```python
from build123d import *

# Parameters (mm, degrees)
SKETCH_1_W          = 40
SKETCH_1_H          = 20
EXTRUDE_1_DEPTH     = 3
EXTRUDE_2_DEPTH     = 3
SKETCH_3_R          = 3
CUT_EXTRUDE_1_DEPTH = 3
SKETCH_4_W          = 40
SKETCH_4_H          = 15
SKETCH_4_R          = 3
EXTRUDE_3_DEPTH     = 3
FILLET_3_R          = 1.5
SKETCH_5_R          = 5
SKETCH_5_R_2        = 3
EXTRUDE_4_DEPTH     = 3
FILLET_4_R          = 1.5
CUT_EXTRUDE_2_DEPTH = 10
FILLET_6_R          = 0.5
CUT_EXTRUDE_3_DEPTH = 3


with BuildPart() as part:
    # 草图1 → 凸台-拉伸1 (new body)
    with BuildSketch(Plane.XY):
        Rectangle(SKETCH_1_W, SKETCH_1_H)
    extrude(amount=EXTRUDE_1_DEPTH)

    # 草图2 → 凸台-拉伸2 (add)
    with BuildSketch(Plane.XY.offset(3)):
        Polygon((-6.9, 8.2), (-6.9, 10), (-13.1, 10), (-13.1, 8.2), (-15.5, 8.2), (-15.5, 6.560660172), (-12.839339828, 3.9), (-7.160660172, 3.9), (-4.5, 6.560660172), (-4.5, 8.2), align=None)
        Polygon((-16.560660172, 5.5), (-18.2, 5.5), (-18.2, 3.1), (-20, 3.1), (-20, -3.1), (-18.2, -3.1), (-18.2, -5.5), (-16.560660172, -5.5), (-13.9, -2.839339828), (-13.9, 2.839339828), align=None)
        Polygon((-12.839339828, -3.9), (-7.160660172, -3.9), (-4.5, -6.560660172), (-4.5, -8.2), (-6.9, -8.2), (-6.9, -10), (-13.1, -10), (-13.1, -8.2), (-15.5, -8.2), (-15.5, -6.560660172), align=None)
        Polygon((18.2, 3.1), (20, 3.1), (20, -3.1), (18.2, -3.1), (18.2, -5.5), (16.560660172, -5.5), (13.9, -2.839339828), (13.9, 2.839339828), (16.560660172, 5.5), (18.2, 5.5), align=None)
        Polygon((13.1, 8.2), (13.1, 10), (6.9, 10), (6.9, 8.2), (4.5, 8.2), (4.5, 6.560660172), (7.160660172, 3.9), (12.839339828, 3.9), (15.5, 6.560660172), (15.5, 8.2), align=None)
        Polygon((7.160660172, -3.9), (12.839339828, -3.9), (15.5, -6.560660172), (15.5, -8.2), (13.1, -8.2), (13.1, -10), (6.9, -10), (6.9, -8.2), (4.5, -8.2), (4.5, -6.560660172), align=None)
    extrude(amount=EXTRUDE_2_DEPTH)

    # 草图3 → 切除-拉伸1 (cut)
    with BuildSketch(Plane(origin=(0, 0, 0), x_dir=(-1, 0, 0), z_dir=(0, 0, -1))):
        with Locations((-10, 0)):
            Circle(SKETCH_3_R)
        with Locations((10, 0)):
            Circle(SKETCH_3_R)
    extrude(amount=-CUT_EXTRUDE_1_DEPTH, mode=Mode.SUBTRACT)

    # 草图4 → 凸台-拉伸3 (add)
    with BuildSketch(Plane(origin=(0, 0, 0), x_dir=(-1, 0, 0), z_dir=(0, 0, -1))):
        with Locations((0, 17.5)):
            Rectangle(SKETCH_4_W, SKETCH_4_H)
        with Locations((-10, 19)):
            Circle(SKETCH_4_R, mode=Mode.SUBTRACT)
        with Locations((10, 19)):
            Circle(SKETCH_4_R, mode=Mode.SUBTRACT)
    extrude(amount=-EXTRUDE_3_DEPTH)

    # 圆角3
    fillet_3_edges = [part.edges().sort_by_distance(p)[0] for p in [
        (20, 25, 1.5),
        (-20, 25, 1.5),
        (20, -10, 1.5),
        (-20, -10, 1.5),
    ]]
    fillet(fillet_3_edges, radius=FILLET_3_R)

    # 草图5 → 凸台-拉伸4 (add)
    # profile 1 of 2: a face of its own
    with BuildSketch(Plane.XY.offset(3)):
        with Locations(Location((-10, 19, 0), (0, 0, 180))):
            Circle(SKETCH_5_R)
        with Locations(Location((-10, 19, 0), (0, 0, 180))):
            Circle(SKETCH_5_R_2, mode=Mode.SUBTRACT)
    # profile 2 of 2: a face of its own
    with BuildSketch(Plane.XY.offset(3)):
        with Locations(Location((10, 19, 0), (0, 0, 180))):
            Circle(SKETCH_5_R)
        with Locations(Location((10, 19, 0), (0, 0, 180))):
            Circle(SKETCH_5_R_2, mode=Mode.SUBTRACT)
    extrude(amount=EXTRUDE_4_DEPTH)

    # 圆角4
    fillet_4_edges = [part.edges().sort_by_distance(p)[0] for p in [
        (-5, 19, 3),
        (15, 19, 3),
    ]]
    fillet(fillet_4_edges, radius=FILLET_4_R)

    # 草图6 → 切除-拉伸2 (cut)
    with BuildSketch(Plane(origin=(0, 0, 0), x_dir=(-1, 0, 0), z_dir=(0, 0, -1))):
        Polygon((0, 23.005790595), (4, 23.005790595), (4, 25), (-4, 25), (-4, 23.005790595), align=None)
        Polygon((0, 15.005790595), (-4, 15.005790595), (-4, 12.005790595), (4, 12.005790595), (4, 15.005790595), align=None)
    extrude(amount=-CUT_EXTRUDE_2_DEPTH, mode=Mode.SUBTRACT)

    # 圆角6
    fillet_6_edges = [part.edges().sort_by_distance(p)[0] for p in [
        (4, 25, 1.5),
        (-4, 25, 1.5),
        (-4, 23.005790595, 1.5),
        (4, 23.005790595, 1.5),
        (4, 12.005790595, 1.5),
        (4, 15.005790595, 1.5),
        (-4, 15.005790595, 1.5),
        (-4, 12.005790595, 1.5),
    ]]
    fillet(fillet_6_edges, radius=FILLET_6_R)

    # 草图7 → 切除-拉伸3 (cut)
    with BuildSketch(Plane.XY.offset(6)):
        Polygon((-18.2, -3.1), (-18.2, -5.5), (-16.560660172, -5.5), (-13.9, -2.839339828), (-13.9, 2.839339828), (-16.560660172, 5.5), (-18.2, 5.5), (-18.2, 3.1), (-20, 3.1), (-20, 2.7), (-19.6, 2.7), (-17.8, 2.7), (-17.8, 5.1), (-16.726345597, 5.1), (-14.3, 2.673654403), (-14.3, -2.673654403), (-16.726345597, -5.1), (-17.8, -5.1), (-17.8, -2.7), (-19.6, -2.7), (-20, -2.7), (-20, -3.1), align=None)
        Polygon((-12.839339828, -3.9), (-15.5, -6.560660172), (-15.5, -8.2), (-13.1, -8.2), (-13.1, -10), (-12.7, -10), (-12.7, -9.6), (-12.7, -7.8), (-15.1, -7.8), (-15.1, -6.726345597), (-12.673654403, -4.3), (-7.326345597, -4.3), (-4.9, -6.726345597), (-4.9, -7.8), (-7.3, -7.8), (-7.3, -9.6), (-7.3, -10), (-6.9, -10), (-6.9, -8.2), (-4.5, -8.2), (-4.5, -6.560660172), (-7.160660172, -3.9), align=None)
        Polygon((-4.5, 8.2), (-6.9, 8.2), (-6.9, 10), (-7.3, 10), (-7.3, 9.6), (-7.3, 7.8), (-4.9, 7.8), (-4.9, 6.726345597), (-7.326345597, 4.3), (-12.673654403, 4.3), (-15.1, 6.726345597), (-15.1, 7.8), (-12.7, 7.8), (-12.7, 9.6), (-12.7, 10), (-13.1, 10), (-13.1, 8.2), (-15.5, 8.2), (-15.5, 6.560660172), (-12.839339828, 3.9), (-7.160660172, 3.9), (-4.5, 6.560660172), align=None)
        Polygon((15.5, 8.2), (13.1, 8.2), (13.1, 10), (12.7, 10), (12.7, 9.6), (12.7, 7.8), (15.1, 7.8), (15.1, 6.726345597), (12.673654403, 4.3), (7.326345597, 4.3), (4.9, 6.726345597), (4.9, 7.8), (7.3, 7.8), (7.3, 9.6), (7.3, 10), (6.9, 10), (6.9, 8.2), (4.5, 8.2), (4.5, 6.560660172), (7.160660172, 3.9), (12.839339828, 3.9), (15.5, 6.560660172), align=None)
        Polygon((18.2, 3.1), (18.2, 5.5), (16.560660172, 5.5), (13.9, 2.839339828), (13.9, -2.839339828), (16.560660172, -5.5), (18.2, -5.5), (18.2, -3.1), (20, -3.1), (20, -2.7), (19.6, -2.7), (17.8, -2.7), (17.8, -5.1), (16.726345597, -5.1), (14.3, -2.673654403), (14.3, 2.673654403), (16.726345597, 5.1), (17.8, 5.1), (17.8, 2.7), (19.6, 2.7), (20, 2.7), (20, 3.1), align=None)
        Polygon((7.160660172, -3.9), (4.5, -6.560660172), (4.5, -8.2), (6.9, -8.2), (6.9, -10), (7.3, -10), (7.3, -9.6), (7.3, -7.8), (4.9, -7.8), (4.9, -6.726345597), (7.326345597, -4.3), (12.673654403, -4.3), (15.1, -6.726345597), (15.1, -7.8), (12.7, -7.8), (12.7, -9.6), (12.7, -10), (13.1, -10), (13.1, -8.2), (15.5, -8.2), (15.5, -6.560660172), (12.839339828, -3.9), align=None)
    extrude(amount=-CUT_EXTRUDE_3_DEPTH, mode=Mode.SUBTRACT)


solid = part.part
```
The model under review builds one solid part; all positions refer to its coordinate system, in mm. A direction names the side the tool comes from. Round coordinates to 2 decimals unless told otherwise and drop trailing zeros. Order: outer loops, then holes, each group sorted by start corner. A loop starts at its lowest first (then second) coordinate and runs counter-clockwise, first axis right, second up. Notation, with made-up numbers: (83, 41.5) -> (92, 41.5) arc R24 cw to (92, 56.5) -> close; hole circle Ø1 at (-26, 4.5). An arc over 180 degrees is marked (long way). One line per item, written item: value. Start each with the question number.
Q1. Take a section at B-B (z = 1.75). Write out the cut boundary in (x, y), and give its area (3 significant figures).
Q2. Clearance check with flat-ended pins moving along their axes: pin 1 Ø2.5 at (x, z) = (5.5, 4.5) entering from -Y; pin 2 Ø0.9 at (x, z) = (-17, 4.5) entering from -Y; pin 3 Ø0.7 at (y, z) = (-8.5, 4) entering from -X. State where each tip first meets the part, or that it passes through.
Q3. Machinability: for faces 5 (the face through (4.9, -7, 5)), 6 (the face through (-15.1, -7, 5)), 7 (the face through (-4, 13, 1)), 8 (the face through (-13.87, 5.496, 4.521)), which of the approach directions +Z, -Z, +X, -X, +Y, -Y give a long, thin tool a straight path to every point of the face, cutting with its end or side? Answer none if there is none.
Q4. Take a section at D-D (x = 10). Count the separate pieces of the cut face and the enclosed holes in it, and give its area (3 significant figures).
Q5. Take a section at C-C (y = 0). Write out the cut boundary in (x, z), and give its area (3 significant figures).
Q6. Wall thickness on line 1 (Y direction, x = -10, z = 1.2); line 2 (X direction, y = 19, z = 5.2); line 3 (Y direction, x = -10, z = 5.25): over which ranges is each line inside the solid? List them lowest first.
Q7. Take a section at A-A (y = 19). Write out the cut boundary in (x, z).
Q8. Mouldability with a two-part tool opening along Y and no side actions: class faces 1 (the face through (-15.53, 3.904, 4.521)), 2 (the face through (-9.9, 22.3, 6)), 3 (the face through (12, 25, 1)), 4 (the face through (4, 14, 1)) as released by +Y, released by -Y, zero draft, split by the parting line, or undercut.
Reported:
1. outline: (-20, -8.5) arc R1.5 ccw to (-18.5, -10) -> (18.5, -10) arc R1.5 ccw to (20, -8.5) -> (20, 23.5) arc R1.5 ccw to (18.5, 25) -> (4.5, 25) arc R0.5 ccw to (4, 24.5) -> (4, 23.51) arc R0.5 cw to (3.5, 23.01) -> (-3.5, 23.01) arc R0.5 cw to (-4, 23.51) -> (-4, 24.5) arc R0.5 ccw to (-4.5, 25) -> (-18.5, 25) arc R1.5 ccw to (-20, 23.5) -> close; hole circle Ø6 at (-10, 0); hole circle Ø6 at (-10, 19); hole (-4, 12.51) arc R0.5 ccw to (-3.5, 12.01) -> (3.5, 12.01) arc R0.5 ccw to (4, 12.51) -> (4, 14.51) arc R0.5 ccw to (3.5, 15.01) -> (-3.5, 15.01) arc R0.5 ccw to (-4, 14.51) -> close; hole circle Ø6 at (10, 0); hole circle Ø6 at (10, 19)
1. area: 1,250 mm2
2. pin 1: stops at y = -7.8
2. pin 2: stops at y = -5.1
2. pin 3: stops at x = -12.7
3. face 5: +Z, -Y
3. face 6: +Z, -X, -Y
3. face 7: +Z, -Z
3. face 8: +Z
4. separate pieces: 3
4. enclosed holes: 0
4. area: 116 mm2
5. outline: (-20, 0) -> (-13, 0) -> (-13, 3) -> (-14.3, 3) -> (-14.3, 6) -> (-20, 6) -> close; (-7, 0) -> (7, 0) -> (7, 3) -> (-7, 3) -> close; (13, 0) -> (20, 0) -> (20, 6) -> (14.3, 6) -> (14.3, 3) -> (13, 3) -> close
5. area: 118 mm2
6. line 1: y = -10 to -3, 3 to 16, 22 to 25
6. line 2: x = -15 to -13, -7 to -5, 5 to 7, 13 to 15
6. line 3: y = -10 to -4.3, 4.3 to 10, 14 to 16, 22 to 24
7. outline: (-20, 0) -> (-13, 0) -> (-13, 6) -> (-15, 6) -> (-15, 4.5) arc R1.5 cw to (-16.5, 3) -> (-20, 3) -> close; (-7, 0) -> (7, 0) -> (7, 6) -> (5, 6) -> (5, 4.5) arc R1.5 cw to (3.5, 3) -> (-3.5, 3) arc R1.5 cw to (-5, 4.5) -> (-5, 6) -> (-7, 6) -> close; (13, 0) -> (20, 0) -> (20, 3) -> (16.5, 3) arc R1.5 cw to (15, 4.5) -> (15, 6) -> (13, 6) -> close
8. face 1: undercut
8. face 2: zero draft
8. face 3: released by +Y
8. face 4: undercut
